Model file for the job. Use its own axes, mm. A direction names the side the tool comes from. Give positions to 0.01 mm unless a question says otherwise; leave off trailing zeros. Write each loop counter-clockwise with the first axis right and the second up, starting at its lowest first coordinate (ties: lowest second). Pieces come first, ordered by that corner, then holes. Notation, with made-up numbers: (42.25, 49) - (85.25, 49) arc R14 cw to (85.25, 53) - close; hole circle Ø11 at (17, 76). An arc over 180 degrees is marked (long way). Use CSV: the item, a comma, the result in double quotes.
from build123d import *

# Parameters (mm, degrees)
SKETCH1_W           = 200
SKETCH1_H           = 180
BOSS_EXTRUDE1_DEPTH = 5
SKETCH3_W           = 20
SKETCH3_H           = 4
CUT_EXTRUDE1_DEPTH  = 5
SKETCH3_6_W         = 20
SKETCH3_6_H         = 4
CUT_EXTRUDE2_DEPTH  = 5
SKETCH3_7_W         = 15
SKETCH3_7_H         = 4
CUT_EXTRUDE3_DEPTH  = 5
SKETCH5_R           = 1.73
CUT_EXTRUDE4_DEPTH  = 5
SKETCH6_W           = 6
SKETCH6_H           = 4
SKETCH6_W_2         = 10
CUT_EXTRUDE5_DEPTH  = 5
SKETCH6_4_W         = 10
SKETCH6_4_H         = 4
SKETCH6_4_W_2       = 6
CUT_EXTRUDE6_DEPTH  = 5
SKETCH7_R           = 1.73
SKETCH7_R_2         = 1.8
CUT_EXTRUDE7_DEPTH  = 5
CUT_EXTRUDE8_DEPTH  = 5
SKETCH9_R           = 1.5
CUT_EXTRUDE11_DEPTH = 5
SKETCH10_R          = 1.73
CUT_EXTRUDE12_DEPTH = 5
SKETCH10_3_R        = 1.73
CUT_EXTRUDE13_DEPTH = 5
SKETCH11_W          = 6
SKETCH11_H          = 6
CUT_EXTRUDE14_DEPTH = 5


with BuildPart() as part:
    # Sketch1 → Boss-Extrude1 (new body)
    with BuildSketch(Plane.XY):
        Rectangle(SKETCH1_W, SKETCH1_H)
    extrude(amount=BOSS_EXTRUDE1_DEPTH)

    # Sketch3 → Cut-Extrude1 (cut)
    with BuildSketch(Plane.XY.offset(5)):
        with Locations((-65, 76)):
            Rectangle(SKETCH3_W, SKETCH3_H)
    cut_extrude1 = extrude(amount=-CUT_EXTRUDE1_DEPTH, mode=Mode.SUBTRACT)

    # Sketch3<6> → Cut-Extrude2 (cut)
    with BuildSketch(Plane.XY.offset(5)):
        with Locations((5, 76)):
            Rectangle(SKETCH3_6_W, SKETCH3_6_H)
    cut_extrude2 = extrude(amount=-CUT_EXTRUDE2_DEPTH, mode=Mode.SUBTRACT)

    # Sketch3<7> → Cut-Extrude3 (cut)
    with BuildSketch(Plane.XY.offset(5)):
        with Locations((72.5, 76)):
            Rectangle(SKETCH3_7_W, SKETCH3_7_H)
    cut_extrude3 = extrude(amount=-CUT_EXTRUDE3_DEPTH, mode=Mode.SUBTRACT)

    # Mirror1: Cut-Extrude1, Cut-Extrude2, Cut-Extrude3 across plane
    add(cut_extrude1.mirror(Plane.ZX), mode=Mode.SUBTRACT)
    add(cut_extrude2.mirror(Plane.ZX), mode=Mode.SUBTRACT)
    add(cut_extrude3.mirror(Plane.ZX), mode=Mode.SUBTRACT)

    # Sketch5 → Cut-Extrude4 (cut)
    with BuildSketch(Plane.XY.offset(5)):
        with Locations((-92, -84)):
            Circle(SKETCH5_R)
        with Locations((-32, -84)):
            Circle(SKETCH5_R)
        with Locations((43, -84)):
            Circle(SKETCH5_R)
        with Locations((76, -84)):
            Circle(SKETCH5_R)
    cut_extrude4 = extrude(amount=-CUT_EXTRUDE4_DEPTH, mode=Mode.SUBTRACT)

    # Mirror2: Cut-Extrude4 across plane
    add(cut_extrude4.mirror(Plane.ZX), mode=Mode.SUBTRACT)

    # Sketch6 → Cut-Extrude5 (cut)
    with BuildSketch(Plane.XY.offset(5)):
        with Locations((-93, 76)):
            Rectangle(SKETCH6_W, SKETCH6_H)
        with Locations((-30, 76)):
            Rectangle(SKETCH6_W_2, SKETCH6_H)
    cut_extrude5 = extrude(amount=-CUT_EXTRUDE5_DEPTH, mode=Mode.SUBTRACT)

    # Sketch6<4> → Cut-Extrude6 (cut)
    with BuildSketch(Plane.XY.offset(5)):
        with Locations((40, 76)):
            Rectangle(SKETCH6_4_W, SKETCH6_4_H)
        with Locations((93, 76)):
            Rectangle(SKETCH6_4_W_2, SKETCH6_4_H)
    cut_extrude6 = extrude(amount=-CUT_EXTRUDE6_DEPTH, mode=Mode.SUBTRACT)

    # Mirror3: Cut-Extrude5, Cut-Extrude6 across plane
    add(cut_extrude5.mirror(Plane.ZX), mode=Mode.SUBTRACT)
    add(cut_extrude6.mirror(Plane.ZX), mode=Mode.SUBTRACT)

    # Sketch7 → Cut-Extrude7 (cut)
    with BuildSketch(Plane.XY.offset(5)):
        with Locations((-82, -84)):
            Circle(SKETCH7_R)
        with Locations((-47, -84)):
            Circle(SKETCH7_R)
        with Locations((8, -84)):
            Circle(SKETCH7_R_2)
        with Locations((60, -84)):
            Circle(SKETCH7_R)
    cut_extrude7 = extrude(amount=-CUT_EXTRUDE7_DEPTH, mode=Mode.SUBTRACT)

    # Mirror4: Cut-Extrude7 across plane
    add(cut_extrude7.mirror(Plane.ZX), mode=Mode.SUBTRACT)

    # Sketch8 → Cut-Extrude8 (cut)
    with BuildSketch(Plane.XY.offset(5)):
        Polygon((0, 45), (25, 45), (25, 55), (0, 55), (-25, 55), (-25, 45), align=None)
    cut_extrude8 = extrude(amount=-CUT_EXTRUDE8_DEPTH, mode=Mode.SUBTRACT)

    # Mirror5: Cut-Extrude8 across plane
    add(cut_extrude8.mirror(Plane.ZX), mode=Mode.SUBTRACT)

    # Sketch9 → Cut-Extrude11 (cut)
    with BuildSketch(Plane.XY.offset(5)):
        with Locations((-3.5, 24.5)):
            Circle(SKETCH9_R)
        with Locations((-61.5, 24.5)):
            Circle(SKETCH9_R)
    cut_extrude11 = extrude(amount=-CUT_EXTRUDE11_DEPTH, mode=Mode.SUBTRACT)

    # Mirror7: Cut-Extrude11 across plane
    add(cut_extrude11.mirror(Plane.ZX), mode=Mode.SUBTRACT)

    # Sketch10 → Cut-Extrude12 (cut)
    with BuildSketch(Plane.XY.offset(5)):
        with Locations((-77.6, -41.875)):
            Circle(SKETCH10_R)
        with Locations((-47.4, -58.125)):
            Circle(SKETCH10_R)
    extrude(amount=-CUT_EXTRUDE12_DEPTH, mode=Mode.SUBTRACT)

    # Sketch10<3> → Cut-Extrude13 (cut)
    with BuildSketch(Plane.XY.offset(5)):
        with Locations((-47.4, 41.88)):
            Circle(SKETCH10_3_R)
        with Locations((-77.6, 58.13)):
            Circle(SKETCH10_3_R)
    extrude(amount=-CUT_EXTRUDE13_DEPTH, mode=Mode.SUBTRACT)

    # Sketch11 → Cut-Extrude14 (cut)
    with BuildSketch(Plane.XY.offset(5)):
        with Locations((-36.5665421, 60)):
            Rectangle(SKETCH11_W, SKETCH11_H)
    cut_extrude14 = extrude(amount=-CUT_EXTRUDE14_DEPTH, mode=Mode.SUBTRACT)

    # Mirror9: Cut-Extrude14 across plane
    add(cut_extrude14.mirror(Plane.ZX), mode=Mode.SUBTRACT)


solid = part.part
(1) Flat gauge pin, fed straight in: P1, Ø1.8, axis at x = -61.5, y = 24.5, coming from the -Z side. Where does the tip first touch, or does it go through?
Checked values:
P1,"passes through"
(2) 3-axis set-ups, long thin cutter, end or side, ignore diameter. For faces 3 (the face through (-39.567, 60, 3)), 4 (the face through (100, -1, 2)): which of +Z, -Z, +X, -X, +Y, -Y reach the whole face in a straight line?
Checked values:
face 3,"+Z, -Z"
face 4,"+Z, -Z, +X, +Y, -Y"
(3) Saw through at A-A, the plane x = -11.5. List the corners of the cut face in (y, z), then the cut area to 3 significant figures.
Checked values:
outline,"(-90, 0) - (-55, 0) - (-55, 5) - (-90, 5) - close; (-45, 0) - (45, 0) - (45, 5) - (-45, 5) - close; (55, 0) - (90, 0) - (90, 5) - (55, 5) - close"
area,"800 mm^2"
(4) Pull direction Y, two halves, no side cores. Call faces 1 (the face through (-1, 1, 5)), 2 (the face through (5, -74, 3)): released by +Y, released by -Y, zero draft, split by the parting line, or undercut.
Checked values:
face 1,"zero draft"
face 2,"undercut"
(5) Saw through at B-B, the plane z = 1.3. Count the separate pieces of the cut face and the enclosed holes in it, then the cut area to 3 significant figures.
Checked values:
separate pieces,"1"
enclosed holes,"42"
area,"34,000 mm^2"
(6) Wall check: probe 1 along Y at (x, z) = (-19.5, 4.15); probe 2 along Y at (x, z) = (-92, 3.35); probe 3 along Y at (x, z) = (67, 4.35). Give the ranges that are in metal, low to high. Write a range as [from, to].
Checked values:
probe 1,"y = [-90, -55], [-45, 45], [55, 90]"
probe 2,"y = [-90, -85.73], [-82.27, -78], [-74, 74], [78, 82.27], [85.73, 90]"
probe 3,"y = [-90, -78], [-74, 74], [78, 90]"
